Autodesk Inventor part; units mm, degrees
ref_plane "YZ Plane" through (0, 0, 0) normal (1, 0, 0) x (0, 1, 0)
ref_plane "XZ Plane" through (0, 0, 0) normal (0, 1, 0) x (-1, 0, 0)
ref_plane "XY Plane" through (0, 0, 0) normal (0, 0, 1) x (1, 0, 0)
sketch "Skizze1" plane through (0, 0, 0) normal (0, 0, 1) x (1, 0, 0)
  line L0 (0, 0) -> (-11.6, 0)
  line L1 (-11.6, 0) -> (-11.6, 1.6)
  line L2 (-11.6, 1.6) -> (-9.6, 1.6)
  line L3 (-9.6, 1.6) -> (-9.6, 4.2)
  line L4 (-9.6, 4.2) -> (-16, 4.2)
  line L5 (-16, 4.2) -> (-16, 7)
  line L6 (-16, 7) -> (0, 7)
  line L7 (0, 7) -> (0, 0)
  dimension "d0" = 9.6
  dimension "d1" = 11.6
  dimension "d2" = 1.6
  dimension "d3" = 4.2
  dimension "d4" = 7
  dimension "d5" = 16
extrude "Extrusion1" add sketch "Skizze1" along normal blind 24
mirror "Spiegeln1" about plane through (0, 0, 0) normal (1, 0, 0) of "Extrusion1"
sketch "Skizze2" plane through (0, 0, 24) normal (0, 0, 1) x (1, 0, 0)
  line L0 (-16, 7) -> (-16, 4.2)
  line L1 (-16, 7) -> (16, 7)
  line L2 (16, 7) -> (16, -5)
  line L3 (16, -5) -> (-16, -5)
  line L4 (-16, -5) -> (-16, 7)
  line L5 (16, 7) -> (16, 4.2)
  point P0 (0, 0)
  dimension "d8" = 12
extrude "Extrusion2" add sketch "Skizze2" along normal blind 5
sketch "Skizze3" plane through (0, 0, 0) normal (1, 0, 0) x (0, 1, 0)
  line L0 (0, 0) -> (0, 24)
  line L1 (0.3, 3.5) -> (1.6, 3.5)
  line L2 (1.6, 3.5) -> (0, 11.5)
  line L3 (0, 11.5) -> (0, 4.0745)
  line L4 (1.6, 0) -> (0, 0)
  line L5 (0.3, 3.5) -> (0.3, 0)
  line L6 (0, 0) -> (0, 4.0745)
  line L7 (-5, 24) -> (4.2, 24)
  point P0 (0, 11.5)
  dimension "d12" = 8
  dimension "d13" = 1.7
  dimension "d14" = 0.3
  dimension "d20" = 20.5
  dimension "d65" = 1.3
extrude "Extrusion3" cut sketch "Skizze3" against normal mid plane 14
sketch "Skizze4" plane through (-16, 7, 0) normal (0, 1, 0) x (1, 0, 0)
  line L0 (3.5, -2) -> (28.5, -2)
  line L1 (28.5, -2) -> (28.5, -29)
  line L2 (28.5, -29) -> (3.5, -29)
  line L3 (3.5, -29) -> (3.5, -2)
  line L4 (16, 0) -> (16, 8.5337)
  line L5 (32, 0) -> (0, 0)
  line L6 (9.5, -26) -> (22.5, -26)
  line L7 (22.5, -26) -> (22.5, -29)
  line L8 (22.5, -29) -> (9.5, -29)
  line L9 (9.5, -29) -> (9.5, -26)
  line L10 (3.5, -29) -> (6.5, -29)
  line L11 (6.5, -29) -> (6.5, -26)
  line L12 (6.5, -26) -> (3.5, -26)
  line L13 (3.5, -26) -> (3.5, -29)
  line L14 (3.5, -2) -> (6.5, -2)
  line L15 (6.5, -2) -> (6.5, -5)
  line L16 (6.5, -5) -> (3.5, -5)
  line L17 (3.5, -5) -> (3.5, -2)
  line L18 (28.5, -29) -> (25.5, -29)
  line L19 (25.5, -29) -> (25.5, -26)
  line L20 (25.5, -26) -> (28.5, -26)
  line L21 (28.5, -26) -> (28.5, -29)
  line L22 (28.5, -2) -> (25.5, -2)
  line L23 (25.5, -2) -> (25.5, -5)
  line L24 (25.5, -5) -> (28.5, -5)
  line L25 (28.5, -5) -> (28.5, -2)
  point P0 (3.5, -26)
  dimension "d17" = 25
  dimension "d18" = 27
  dimension "d19" = 2
  dimension "d21" = 3
  dimension "d22" = 13
  dimension "d23" = 24
  dimension "d24" = 3
  dimension "d25" = 3
  dimension "d26" = 3
  dimension "d27" = 3
  dimension "d28" = 3
  dimension "d29" = 3
  dimension "d30" = 3
  dimension "d31" = 3
extrude "Extrusion4" cut sketch "Skizze4" against normal blind 1 contours L0 L23 L24 L1 L20 L19 L2 L7 L6 L9 L11 L12 L3 L16 L15
extrude "Extrusion5" cut sketch "Skizze4" against normal blind 10 contours L9 L6 L7 L2
sketch "Skizze5" plane through (0, 0, 29) normal (0, 0, 1) x (1, 0, 0)
  circle A0 centre (12, -1) radius 1.75
  line L0 (-16, -5) -> (16, -5)
  line L1 (16, -5) -> (16, 7)
  point P0 (0, 0)
  dimension "d36" = 3.5
  dimension "d37" = 4
  dimension "d38" = 4
extrude "Extrusion6" cut sketch "Skizze5" against normal blind 6.75
sketch "Skizze6" plane through (0, 0, 24) normal (0, 0, -1) x (-1, 0, 0)
  arc A0 (-11.6, 0.7037) -> (-10.5639, 0) centre (-12, -1) ccw
  line L0 (-10.2968, -3.95) -> (-13.7032, -3.95)
  line L1 (-13.7032, -3.95) -> (-15.4064, -1)
  line L2 (-15.4064, -1) -> (-13.7032, 1.95)
  line L3 (-13.7032, 1.95) -> (-10.2968, 1.95)
  line L4 (-10.2968, 1.95) -> (-8.5936, -1)
  line L5 (-8.5936, -1) -> (-10.2968, -3.95)
  point P0 (0, 0)
  dimension "d42" = 5.9
extrude "Extrusion7" cut sketch "Skizze6" along normal mid plane 7.5
sketch "Skizze7" plane through (16, 4.2, 0) normal (1, 0, 0) x (0, 0, -1)
  line L0 (-29, 1.8) -> (-29, -7.2)
  circle A0 centre (-29, -0.2) radius 2
  line L1 (0, 2.8) -> (-29, 2.8)
  point P0 (0, -4.2)
  point P1 (-29, -2.2)
  dimension "d45" = 4
  dimension "d46" = 3
extrude "Extrusion8" cut sketch "Skizze7" against normal blind 10 contours A0 L0 picked at (-28.3333, -0.2)
sketch "Skizze9" plane through (16, 4.2, 0) normal (1, 0, 0) x (0, 0, -1)
  line L0 (0, 0) -> (-24, 0)
  line L1 (0, 0) -> (-1, 0)
  line L2 (-1, 0) -> (-1, 1.6)
  line L3 (-1, 1.6) -> (0, 1.6)
  line L4 (0, 1.6) -> (0, 0)
  line L5 (0, 2.8) -> (-29, 2.8)
  line L6 (0, 2.8) -> (0, 0)
  line L7 (0, 2.8) -> (-0.2, 2.8)
  line L8 (-0.2, 2.8) -> (-0.2, 1.6)
  line L9 (-0.2, 1.6) -> (0, 1.6)
  line L10 (0, 1.6) -> (0, 2.8)
  point P0 (0, -4.2)
  dimension "d60" = 1
  dimension "d61" = 1.2
  dimension "d62" = 0.2
extrude "Extrusion10" cut sketch "Skizze9" against normal up to surface (32 mm away)
fillet "Rundung1" radius 2.5 1 edges at (16, -5, 26.5)
fillet "Rundung2" radius 4 1 edges at (-16, -5, 26.5)
equation "\"d38\" = d37"
properties part number "DisplayClipLower"
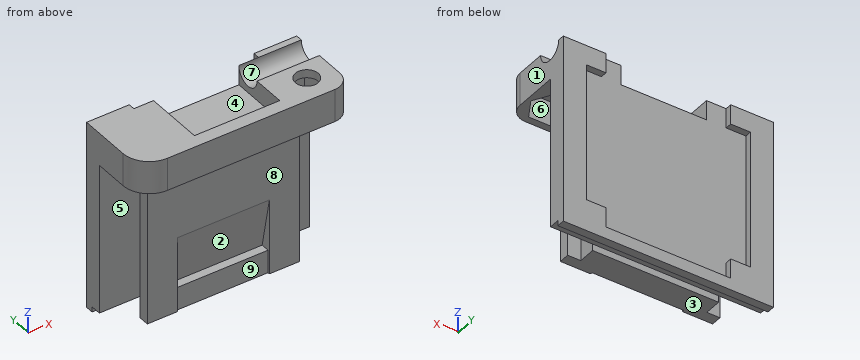
The model under review builds one solid part; all positions refer to its coordinate system, in mm. Face numbers are marked on the shaded views. A direction names the side the tool comes from. Round coordinates to 2 decimals unless told otherwise and drop trailing zeros. Order: outer loops, then holes, each group sorted by start corner. A loop starts at its lowest first (then second) coordinate and runs counter-clockwise, first axis right, second up. Notation, with made-up numbers: (-21, -4.75) - (20, -4.75) arc R20 cw to (20, 9.25) - close; hole circle Ø6 at (37, 61). An arc over 180 degrees is marked (long way). Answer in a Markdown table with one row per item.
(1) Clearance check with flat-ended pins moving along their axes: P1, Ø0.5, axis at y = 0.5, z = 6.5, coming from the -X side; P2, Ø1, axis at x = -10, z = 8, coming from the +Y side; P3, Ø1.1, axis at x = 4, y = 6.5, coming from the +Z side. State where each tip first meets the part, or that it passes through.
Result set:
| item | result |
|---|---|
| P1 | stops at x = -11.6 |
| P2 | stops at y = 6 |
| P3 | stops at z = 26 |
(2) Take a section at C-C on z = 15.25. Write out the cut boundary in (x, y), plus the area to 3 significant figures.
Result set:
| item | result |
|---|---|
| outline | (-16, 4.2) - (-9.6, 4.2) - (-9.6, 1.6) - (-11.6, 1.6) - (-11.6, 0) - (11.6, 0) - (11.6, 1.6) - (9.6, 1.6) - (9.6, 4.2) - (16, 4.2) - (16, 7) - (12.5, 7) - (12.5, 6) - (-12.5, 6) - (-12.5, 7) - (-16, 7) - close |
| area | 152 mm2 |
(3) For line 1 (Y direction, x = 12, z = 28.6); line 2 (Y direction, x = 12, z = 28.35); line 3 (Z direction, x = 9.5, y = -3), list the stretches that pass through material, from the lowest coordinate up. Write a range as from..to.
Result set:
| item | result |
|---|---|
| line 1 | y = -5..-2.75, 0.75..2.04, 5.96..7 |
| line 2 | y = -5..-2.75, 0.75..2.11, 5.89..7 |
| line 3 | z = 24..29 |
(4) Mouldability with a two-part tool opening along X and no side actions: class the marked faces 1, 2, 3 and 4 as released by +X, released by -X, zero draft, split by the parting line, or undercut.
Result set:
| item | result |
|---|---|
| face 1 | released by +X |
| face 2 | undercut |
| face 3 | zero draft |
| face 4 | undercut |
(5) Take a section at D-D on x = -10. Write out the cut boundary in (y, z), plus the area to 3 significant figures.
Result set:
| item | result |
|---|---|
| outline | (-5, 24) - (0, 24) - (0, 0) - (1.6, 0) - (1.6, 24) - (4.2, 24) - (4.2, 1) - (5.8, 1) - (5.8, 0.2) - (7, 0.2) - (7, 5) - (6, 5) - (6, 26) - (7, 26) - (7, 29) - (-5, 29) - close |
| area | 143 mm2 |
(6) Take a section at A-A on x = 12. Write out the cut boundary in (y, z), plus the area to 3 significant figures.
Result set:
| item | result |
|---|---|
| outline | (-5, 24) - (-3.95, 24) - (-3.95, 27.75) - (-2.75, 27.75) - (-2.75, 29) - (-5, 29) - close; (0.75, 27.75) - (1.95, 27.75) - (1.95, 24) - (4.2, 24) - (4.2, 1) - (5.8, 1) - (5.8, 0.2) - (7, 0.2) - (7, 5) - (6, 5) - (6, 26) - (7, 26) - (7, 29) - (6, 29) arc R2 cw to (2, 29) - (0.75, 29) - close |
| area | 71.6 mm2 |
(7) Take a section at B-B on y = -0.5. Write out the cut boundary in (x, z), plus the area to 3 significant figures.
Result set:
| item | result |
|---|---|
| outline | (-16, 24) - (8.88, 24) - (8.88, 27.75) - (10.32, 27.75) - (10.32, 29) - (6.5, 29) - (6.5, 26) - (-6.5, 26) - (-6.5, 29) - (-16, 29) - close; (13.68, 27.75) - (15.12, 27.75) - (15.12, 24) - (16, 24) - (16, 29) - (13.68, 29) - close |
| area | 93.4 mm2 |
(8) Machinability: for the marked faces 5, 6, 7, 8 and 9, which of the approach directions +Z, -Z, +X, -X, +Y, -Y give a long, thin tool a straight path to every point of the face, cutting with its end or side? Answer none if there is none.
Result set:
| item | result |
|---|---|
| face 5 | -Z, -X |
| face 6 | -Z |
| face 7 | +Z, +X |
| face 8 | -Z, +X, -X, -Y |
| face 9 | -Z, -Y |
